Read the model definition and answer for the solid it produces. Units are mm, in the model's axes. A direction names the side the tool comes from. Give positions to 0.01 mm unless a question says otherwise; leave off trailing zeros. Order: outer loops, then holes, each group sorted by start corner. A loop starts at its lowest first (then second) coordinate and runs counter-clockwise, first axis right, second up. Notation, with made-up numbers: (-22, 61) -> (-11, 61) arc R22 cw to (-11, 88) -> close; hole circle Ø1 at (-17.5, -10). An arc over 180 degrees is marked (long way). One line per question, with ' | ' between items. Start each with the question number.
```python
from build123d import *

# Parameters (mm, degrees)
SKETCH2_W                             = 76.2
SKETCH2_H                             = 50.8
BOSS_EXTRUDE1_DEPTH                   = 25.4
TAP_DRILL_FOR_1_4_20_TAP1_AT_2_COUNT  = 2
TAP_DRILL_FOR_1_4_20_TAP1_AT_2_PITCH  = 22.895250599
TAP_DRILL_FOR_1_4_20_TAP1_AT_3_COUNT  = 2
TAP_DRILL_FOR_1_4_20_TAP1_AT_3_PITCH  = 38.1
F_3_32_0_09375_DOWEL_HOLE1_AT_2_COUNT = 2
F_3_32_0_09375_DOWEL_HOLE1_AT_2_PITCH = 38.1
F_3_32_0_09375_DOWEL_HOLE1_AT_3_COUNT = 2
F_3_32_0_09375_DOWEL_HOLE1_AT_3_PITCH = 22.895250599
CUT_EXTRUDE1_DEPTH                    = 53.363441445


with BuildPart() as part:
    # Sketch2 → Boss-Extrude1 (new body)
    with BuildSketch(Plane.XY):
        Rectangle(SKETCH2_W, SKETCH2_H)
    extrude(amount=BOSS_EXTRUDE1_DEPTH)

    # Sketch6 → Tap Drill for 1/4-20 Tap1 (revolve, cut)
    with BuildSketch(Plane(origin=(-38.1, 19.05, 19.05), x_dir=(0, 0, 1), z_dir=(0, 1, 0))):
        Polygon((0, 0), (0, 20.583816902), (2.5527, 19.05), (2.5527, 0), align=None)
    tap_drill_for_1_4_20_tap1 = revolve(axis=Axis((-44.45, 19.05, 19.05), (1, 0, 0)), mode=Mode.SUBTRACT)

    # Tap Drill for 1/4-20 Tap1 at 2: Tap Drill for 1/4-20 Tap1 ×2
    with Locations(*[Vector(2.831898447985745e-15, -0.8320502943378457, -0.554700196225226) * (i * TAP_DRILL_FOR_1_4_20_TAP1_AT_2_PITCH) for i in range(1, TAP_DRILL_FOR_1_4_20_TAP1_AT_2_COUNT)]):
        add(tap_drill_for_1_4_20_tap1, mode=Mode.SUBTRACT)

    # Tap Drill for 1/4-20 Tap1 at 3: Tap Drill for 1/4-20 Tap1 ×2
    with Locations(*[(0, -i * TAP_DRILL_FOR_1_4_20_TAP1_AT_3_PITCH, 0) for i in range(1, TAP_DRILL_FOR_1_4_20_TAP1_AT_3_COUNT)]):
        add(tap_drill_for_1_4_20_tap1, mode=Mode.SUBTRACT)

    # Sketch8 → 3/32 (0.09375) Dowel Hole1 (revolve, cut)
    with BuildSketch(Plane(origin=(-38.1, 19.05, 6.35), x_dir=(0, 0, 1), z_dir=(0, 1, 0))):
        Polygon((0, 0), (0, 8.652899675), (1.190625, 7.9375), (1.190625, 0), align=None)
    f_3_32_0_09375_dowel_hole1 = revolve(axis=Axis((-44.45, 19.05, 6.35), (1, 0, 0)), mode=Mode.SUBTRACT)

    # 3/32 (0.09375) Dowel Hole1 at 2: 3/32 (0.09375) Dowel Hole1 ×2
    with Locations(*[(0, -i * F_3_32_0_09375_DOWEL_HOLE1_AT_2_PITCH, 0) for i in range(1, F_3_32_0_09375_DOWEL_HOLE1_AT_2_COUNT)]):
        add(f_3_32_0_09375_dowel_hole1, mode=Mode.SUBTRACT)

    # 3/32 (0.09375) Dowel Hole1 at 3: 3/32 (0.09375) Dowel Hole1 ×2
    with Locations(*[Vector(2.831898447985753e-15, -0.8320502943378447, 0.5547001962252276) * (i * F_3_32_0_09375_DOWEL_HOLE1_AT_3_PITCH) for i in range(1, F_3_32_0_09375_DOWEL_HOLE1_AT_3_COUNT)]):
        add(f_3_32_0_09375_dowel_hole1, mode=Mode.SUBTRACT)

    # Mirror1: Tap Drill for 1/4-20 Tap1, 3/32 (0.09375) Dowel Hole1 across plane
    add(tap_drill_for_1_4_20_tap1.mirror(Plane(origin=(0, 0, 0), x_dir=(0, 0, 1), z_dir=(1, 0, 0))), mode=Mode.SUBTRACT)
    add(f_3_32_0_09375_dowel_hole1.mirror(Plane(origin=(0, 0, 0), x_dir=(0, 0, 1), z_dir=(1, 0, 0))), mode=Mode.SUBTRACT)

    # Mirror1 copy 1 sketch → Mirror1 copy 1 (revolve, cut)
    with BuildSketch(Plane(origin=(38.1, 0, 6.35), x_dir=(0, 0, 1), z_dir=(0, 1, 0))):
        Polygon((0, 0), (0, -20.583816902), (2.5527, -19.05), (2.5527, 0), align=None)
    revolve(axis=Axis((44.45, 0, 6.35), (1, 0, 0)), mode=Mode.SUBTRACT)

    # Mirror1 copy 2 sketch → Mirror1 copy 2 (revolve, cut)
    with BuildSketch(Plane(origin=(38.1, -19.05, 19.05), x_dir=(0, 0, 1), z_dir=(0, 1, 0))):
        Polygon((0, 0), (0, -20.583816902), (2.5527, -19.05), (2.5527, 0), align=None)
    revolve(axis=Axis((44.45, -19.05, 19.05), (1, 0, 0)), mode=Mode.SUBTRACT)

    # Mirror1 copy 3 sketch → Mirror1 copy 3 (revolve, cut)
    with BuildSketch(Plane(origin=(38.1, -19.05, 6.35), x_dir=(0, 0, 1), z_dir=(0, 1, 0))):
        Polygon((0, 0), (0, -8.652899675), (1.190625, -7.9375), (1.190625, 0), align=None)
    revolve(axis=Axis((44.45, -19.05, 6.35), (1, 0, 0)), mode=Mode.SUBTRACT)

    # Mirror1 copy 4 sketch → Mirror1 copy 4 (revolve, cut)
    with BuildSketch(Plane(origin=(38.1, 0, 19.05), x_dir=(0, 0, 1), z_dir=(0, 1, 0))):
        Polygon((0, 0), (0, -8.652899675), (1.190625, -7.9375), (1.190625, 0), align=None)
    revolve(axis=Axis((44.45, 0, 19.05), (1, 0, 0)), mode=Mode.SUBTRACT)

    # Sketch4 → Cut-Extrude1 (cut, through all)
    with BuildSketch(Plane(origin=(0, 0, 0), x_dir=(-1, 0, 0), z_dir=(0, 0, -1))):
        Polygon((3.666174209, 6.35), (-3.666174209, 6.35), (-7.332348419, 0), (-3.666174209, -6.35), (3.666174209, -6.35), (7.332348419, 0), align=None)
    extrude(amount=-CUT_EXTRUDE1_DEPTH, mode=Mode.SUBTRACT)


solid = part.part
```
Q1. Which of the six approach directions +Z, -Z, +X, -X, +Y, -Y give full straight-line access (tool end or side, diameter ignored) to faces 1 (the cylindrical face through (-34.19, 17.87, 6.2)), 2 (the flat face through (-5.525, 3.131, 12.522)), 3 (the flat face through (-1, -25.4, 13)), 4 (the flat face through (8, 0, 0)), 5 (the cylindrical face through (34.19, 17.87, 6.2))?
Q2. Find the intervals of material crossed by line 1 (Y direction, x = 26, z = 19.05); line 2 (Y direction, x = 35.25, z = 19.05); line 3 (Z direction, x = 35.5, y = -19.05), in increasing order.
Q3. A cutting plane is placed at A-A, the plane z = 13. Determine the outline of the cut face in (x, y).
Q4. Given P1, Ø1.9, axis at y = 19.05, z = 6.35, coming from the -X side; P2, Ø3, axis at y = 19.05, z = 19.05, coming from the -X side; P3, Ø2, axis at y = 0, z = 19.05, coming from the +X side, each flat-ended and moving along its own axis, determine where each tip first touches the part or whether it passes through.
Q5. Determine the mould class of faces 6 (the conical face through (-29.57, 0.08, 19.24)), 7 (the flat face through (-1, 25.4, 13)), 8 (the flat face through (-38.1, 0, 13)), 9 (the cylindrical face through (-28.708, -16.558, 18.497)) for opening direction Y: pulls with the +Y half, pulls with the -Y half, needs draft (parallel to the pull), parting line crosses it, or undercut.
Geometry results:
1) face 1: -X | face 2: +Z, -Z | face 3: +Z, -Z, +X, -X, -Y | face 4: -Z, +X, -X, +Y, -Y | face 5: +X
2) line 1: -25.4 to -21.6, -16.5 to 16.5, 21.6 to 25.4 | line 2: -25.4 to -21.6, -16.5 to -1.19, 1.19 to 16.5, 21.6 to 25.4 | line 3: 0 to 5.16, 7.54 to 16.5, 21.6 to 25.4
3) outline: (-38.1, -25.4) -> (38.1, -25.4) -> (38.1, 25.4) -> (-38.1, 25.4) -> close; hole (-7.33, 0) -> (-3.67, -6.35) -> (3.67, -6.35) -> (7.33, 0) -> (3.67, 6.35) -> (-3.67, 6.35) -> close
4) P1: x = -30.02 | P2: x = -18.42 | P3: x = 30.05
5) face 6: undercut | face 7: pulls with the +Y half | face 8: needs draft | face 9: undercut
